Input: dimensioned drawing with shaded views. Units: mm. Origin: part minimum x, y, z. Coordinates: 2 decimals unless noted, no trailing zeros. Loops run counter-clockwise (first coordinate to the right, second up) from the corner with the lowest first, then second, coordinate; pieces in that order, holes last. Notation, with made-up numbers: (-7, 81) -> (27, 81) arc R17 cw to (27, 103) -> close; hole circle Ø8 at (18.5, 48). An arc over 180 degrees is marked (long way). Answer as CSV lines item,"result".
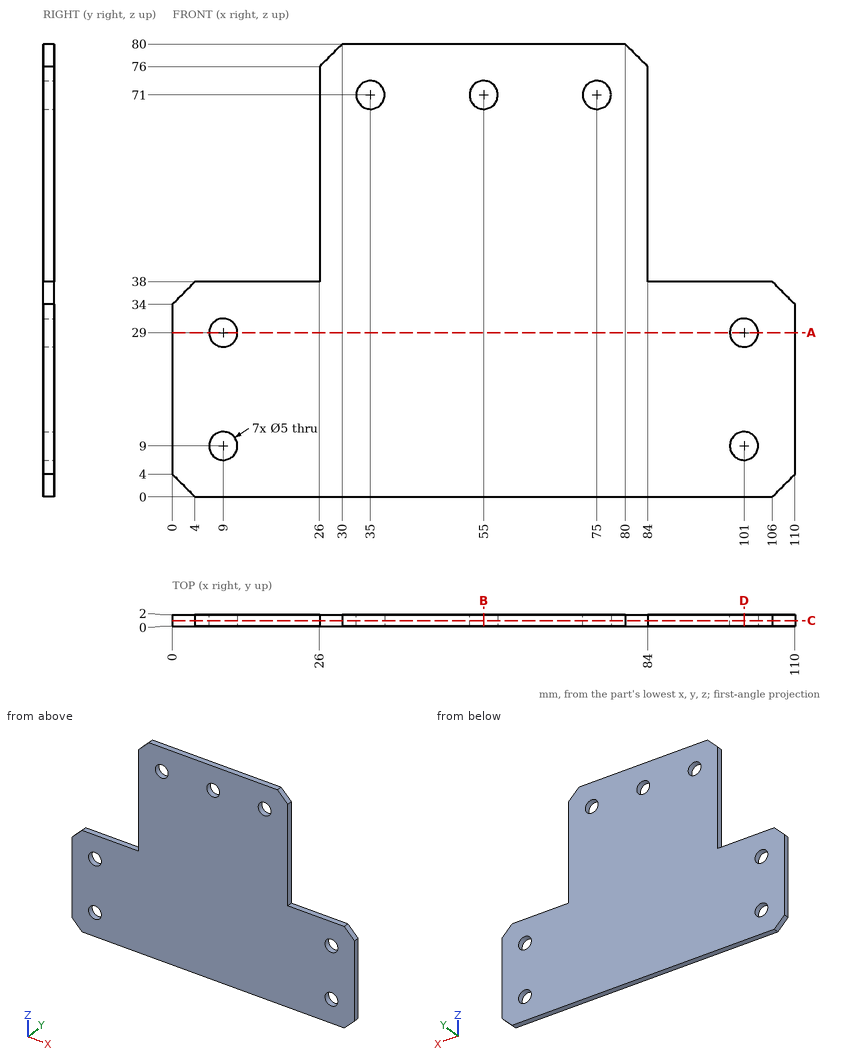
(1) Pin query (flat end, axial travel): pin 1 Ø4.5 at (x, z) = (55, 71) entering from +Y; pin 2 Ø1 at (y, z) = (1.5, 66) entering from +X; pin 3 Ø1 at (x, y) = (94, 1.5) entering from +Z; pin 4 Ø1 at (y, z) = (1, 64.5) entering from -X. Return the tip coordinate at first contact, or that it passes through.
Computed values:
pin 1,"through"
pin 2,"x = 84"
pin 3,"z = 38"
pin 4,"x = 26"
(2) Material intervals for L1, parallel to Z at x = 9, y = 1.1; L2, parallel to Z at x = 55, y = 1.4; L3, parallel to X at y = 0.4, z = 28, sorted ascending. Write a range as [from, to].
Computed values:
L1,"[0, 6.5], [11.5, 26.5], [31.5, 38]"
L2,"[0, 68.5], [73.5, 80]"
L3,"[0, 6.71], [11.29, 98.71], [103.29, 110]"
(3) Cut plane C-C (y = 1). Return the cut outline in (x, z), then the cut area to 3 significant figures.
Computed values:
outline,"(0, 4) -> (4, 0) -> (106, 0) -> (110, 4) -> (110, 34) -> (106, 38) -> (84, 38) -> (84, 76) -> (80, 80) -> (30, 80) -> (26, 76) -> (26, 38) -> (4, 38) -> (0, 34) -> close; hole circle Ø5 at (9, 9); hole circle Ø5 at (9, 29); hole circle Ø5 at (35, 71); hole circle Ø5 at (55, 71); hole circle Ø5 at (75, 71); hole circle Ø5 at (101, 9); hole circle Ø5 at (101, 29)"
area,"6,430 mm^2"
(4) Cut plane D-D (x = 101). Return the cut outline in (y, z), then the cut area to 3 significant figures.
Computed values:
outline,"(0, 0) -> (2, 0) -> (2, 6.5) -> (0, 6.5) -> close; (0, 11.5) -> (2, 11.5) -> (2, 26.5) -> (0, 26.5) -> close; (0, 31.5) -> (2, 31.5) -> (2, 38) -> (0, 38) -> close"
area,"56.0 mm^2"
(5) Cut plane A-A (z = 29). Return the cut outline in (x, y).
Computed values:
outline,"(0, 0) -> (6.5, 0) -> (6.5, 2) -> (0, 2) -> close; (11.5, 0) -> (98.5, 0) -> (98.5, 2) -> (11.5, 2) -> close; (103.5, 0) -> (110, 0) -> (110, 2) -> (103.5, 2) -> close"
(6) Cut plane B-B (x = 55). Return the cut outline in (y, z), then the cut area to 3 significant figures.
Computed values:
outline,"(0, 0) -> (2, 0) -> (2, 68.5) -> (0, 68.5) -> close; (0, 73.5) -> (2, 73.5) -> (2, 80) -> (0, 80) -> close"
area,"150 mm^2"
